Check sheet for the modelled part. Datum: model origin and axes. Units: mm. Give positions to 0.01 mm unless a question says otherwise; leave off trailing zeros. Loops run counter-clockwise (first coordinate to the right, second up) from the corner with the lowest first, then second, coordinate; pieces in that order, holes last. Notation, with made-up numbers: M -15.5,54 L 10.5,54 A24 ccw 10.5,91 Z; hole C 28,80 d9. An arc over 180 degrees is marked long. One line per question, with ' | ' between items. Start each with the question number.
from build123d import *

# Parameters (mm, degrees)
BOSS_EXTRUDE1_DEPTH = 3


with BuildPart() as part:
    # Sketch1 → Boss-Extrude1 (new body)
    with BuildSketch(Plane(origin=(0, 0, 0), x_dir=(1, 0, 0), z_dir=(0, 1, 0))):
        with BuildLine():
            Line((-31.5, 0), (-31.5, -23.5))
            ThreePointArc((-31.5, -23.5), (0, -55), (31.5, -23.5))
            Line((31.5, -23.5), (31.5, -3))
            Line((31.5, -3), (31.8, -3))
            Line((31.8, -3), (31.8, -23.5))
            ThreePointArc((31.8, -23.5), (0, -55.3), (-31.8, -23.5))
            Line((-31.8, -23.5), (-31.8, 0))
            Line((-31.8, 0), (-31.5, 0))
        make_face()
    extrude(amount=BOSS_EXTRUDE1_DEPTH)


solid = part.part
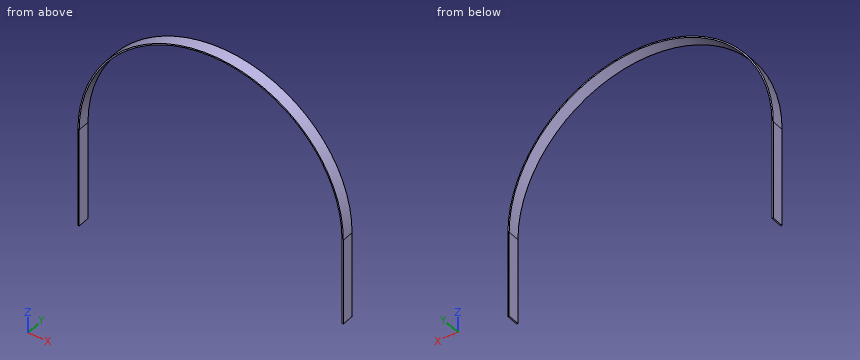
Q1. Material ranges on probe 1 along X at (y, z) = (1.4, 20); probe 2 along X at (y, z) = (0.3, 41); probe 3 along Z at (x, y) = (0, 2.8), recorded low to high. Write a range as from..to.
Q2. Cross-section at D-D (z = 22.5). Record the cut outline in (x, y).
Q3. Depth check by flat-ended pin: P1, Ø1.5, axis at x = -4, y = 2, coming from the +Z side. Enter the tip coordinate at first touch or a pass-through.
Q4. Cross-section at C-C (x = 0). Record the cut outline in (y, z).
Q5. Cross-section at B-B (y = 1.25). Record the cut outline in (x, z), and give its area (3 significant figures).
Solved:
1) probe 1: x = -31.8..-31.5, 31.5..31.8 | probe 2: x = -26.55..-26.19, 26.19..26.55 | probe 3: z = 55..55.3
2) outline: M -31.8,0 L -31.5,0 L -31.5,3 L -31.8,3 Z; M 31.5,0 L 31.8,0 L 31.8,3 L 31.5,3 Z
3) P1: stops at z = 55.13
4) outline: M 0,55 L 3,55 L 3,55.3 L 0,55.3 Z
5) outline: M -31.8,0 L -31.5,0 L -31.5,23.5 A31.5 cw 31.5,23.5 L 31.5,3 L 31.8,3 L 31.8,23.5 A31.8 ccw -31.8,23.5 Z | area: 43.0 mm²
